from build123d import *

# Parameters (mm, degrees)
F5_COUNT = 4
F6_R     = 7.62
F7_R     = 5.08
F8_R     = 5.08


with BuildPart() as f1:
    # F0 (on Front) → F1 (revolve)
    with BuildSketch(Plane.XZ):
        Polygon((-30.2196051925, 0), (0, 0), (0, 21.5392599132), (-22.1149149458, 21.5392599132), (-22.1149149458, 6.6195321269), (-30.2196051925, 6.6195321269), align=None)
    revolve(axis=Axis((0, 0, 62.8589570214), (0, 0, 1)))



with BuildPart() as f1b:
    # F0 (on Front) → F1, piece 2 (revolve)
    with BuildSketch(Plane.XZ):
        with BuildLine():
            Line((-22.1149149458, 47.1819389861), (0, 47.1819389861))
            Line((0, 47.1819389861), (0, 78.5359750567))
            ThreePointArc((0, 78.5359750567), (-13.2981646967, 69.5796959287), (-9.9974415372, 53.8901660841))
            Line((-9.9974415372, 53.8901660841), (-22.1149149458, 47.1819389861))
        make_face()
    revolve(axis=Axis((0, 0, 62.8589570214), (0, 0, 1)))


with BuildPart() as f1_1:
    add(f1.part)

    add(f1b.part)  # F4 merges F1b
    # F3 (on face) → F4 section 0
    with BuildSketch(Plane(origin=(0, 0, 47.1819389861), x_dir=(1, 0, 0), z_dir=(0, 0, -1))):
        with BuildLine():
            Line((-15.7649149458, 0), (-21.1836484832, 6.35))
            ThreePointArc((-21.1836484832, 6.35), (-22.1149149458, 0), (-21.1836484832, -6.35))
            Line((-21.1836484832, -6.35), (-15.7649149458, 0))
        make_face()
    # F2 (on face) → F4 section 1
    with BuildSketch(Plane.XY.offset(21.5392599132)):
        with BuildLine():
            Line((0, -15.7649149458), (-6.35, -21.1836484832))
            ThreePointArc((-6.35, -21.1836484832), (0, -22.1149149458), (6.35, -21.1836484832))
            Line((6.35, -21.1836484832), (0, -15.7649149458))
        make_face()
    loft()

    # F5: F1 ×4 about axis
    f5_axis = Axis((0, 0, 21.5392599132), (0, 0, 1))


with BuildPart() as f1_2:
    add(f1_1.part)
    for i in range(1, F5_COUNT):
        add(f1_1.part.rotate(f5_axis, i * 360 / F5_COUNT))

    # F6
    f6_edges = [f1_2.edges().sort_by_distance(p)[0] for p in [
        (22.114915, 0, 6.619532),
    ]]
    fillet(f6_edges, radius=F6_R)

    # F7
    f7_edges = [f1_2.edges().sort_by_distance(p)[0] for p in [
        (30.219605, 0, 6.619532),
    ]]
    fillet(f7_edges, radius=F7_R)

    # F8
    f8_edges = [f1_2.edges().sort_by_distance(p)[0] for p in [
        (9.997442, 0, 53.890166),
    ]]
    fillet(f8_edges, radius=F8_R)


solid = f1_2.part
Input: part model. Units: mm. Frame: model coordinates. Coordinates: 2 decimals unless noted, no trailing zeros. Order: outer loops, then holes, each group sorted by start corner. A loop starts at its lowest first (then second) coordinate and runs counter-clockwise, first axis right, second up. Notation, with made-up numbers: M -32.75,32.25 L -7.75,32.25 A9 ccw -7.75,40.25 Z; hole C 84.25,-6.5 d6. An arc over 180 degrees is marked long. Write item = value, one per line. Start each with the question number.
(1) Section D-D on z = 17. Output: boundary loops of the cut face in (x, y).
(2) Section A-A on x = 9.5. Give the number of separate pieces and of enclosed holes in the cut face, and give its area (3 significant figures).
(3) Pull-direction query (Y, two-part tool) for faces 1 (the flat face through (0, 0, 47.182)), 2 (the flat face through (0, 0, 21.539)), 3 (the flat face through (0, 0, 0)), 4 (the cylindrical face through (4.79, 21.59, 17.84)); classes: released by +Y, released by -Y, zero draft, split by the parting line, or undercut.
(4) First-contact query: P1, Ø2, axis at x = 1.5, y = 8, coming from the +Z side; P2, Ø12, axis at y = 4.5, z = 41.5, coming from the +X side; P3, Ø1.5, axis at y = 12, z = 54.5, coming from the +X side. Flat tips, straight axial feed; report the tip coordinate or a pass-through.
(5) Line query: line 1 along Z through (x, y) = (11.5, 10.5); line 2 along Z through (x, y) = (16, 0); line 3 along Z through (x, y) = (-5.5, -4.5). Output: solid intervals per line, ascending. Write a range as [from, to].
Result set:
q1.outline = C 0,0 d44.23
q2.separate_pieces = 4
q2.enclosed_holes = 0
q2.area = 1,660 mm²
q3.face_1 = undercut
q3.face_2 = undercut
q3.face_3 = zero draft
q3.face_4 = split by the parting line
q4.P1 = 76.63
q4.P2 = 21.96
q4.P3 = 5.41
q5.line_1 = [0, 21.54], [32.75, 37.34], [47.18, 50.8]
q5.line_2 = [0, 28.13], [40.59, 50.57]
q5.line_3 = [0, 21.54], [47.18, 76.65]
